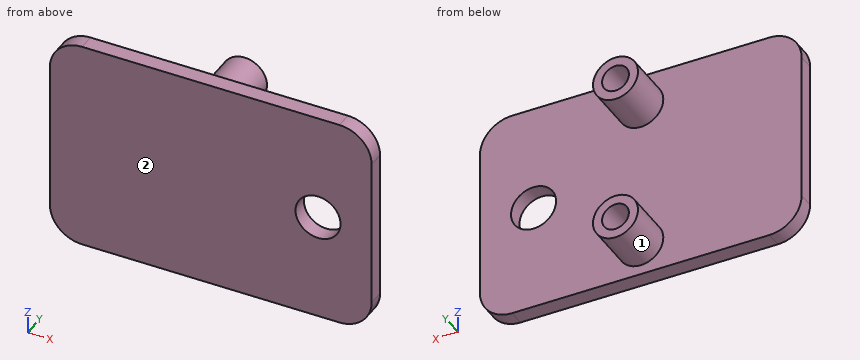
```python
from build123d import *

# Parameters (mm, degrees)
SKETCH_1_R             = 2.1
SM_BASE_FLANGE_1_DEPTH = 1.5
SKETCH_2_R             = 2.1
EXTRUDE_1_DEPTH        = 4.5
HOLE_WIZARD_M3_1_D     = 2.5
HOLE_WIZARD_M3_1_DEPTH = 4


# Sheet-metal steps are written as plain solids
with BuildPart() as part:
    # Sketch 1 → 基体-法兰1 (new body)
    with BuildSketch(Plane(origin=(0, 0, 0), x_dir=(1, 0, 0), z_dir=(0, 1, 0))):
        with BuildLine():
            Line((-7.384325118, 10), (16.615674882, 10))
            ThreePointArc((16.615674882, 10), (18.736995226, 9.121320344), (19.615674882, 7))
            Line((19.615674882, 7), (19.615674882, -7))
            ThreePointArc((19.615674882, -7), (18.736995226, -9.121320344), (16.615674882, -10))
            Line((16.615674882, -10), (-7.384325118, -10))
            ThreePointArc((-7.384325118, -10), (-9.505645461, -9.121320344), (-10.384325118, -7))
            Line((-10.384325118, -7), (-10.384325118, 7))
            ThreePointArc((-10.384325118, 7), (-9.505645461, 9.121320344), (-7.384325118, 10))
        make_face()
        with Locations(Location((14.615674882, 0, 0), (0, 0, 270))):
            Circle(SKETCH_1_R, mode=Mode.SUBTRACT)
    extrude(amount=-SM_BASE_FLANGE_1_DEPTH)

    # Sketch 2 → 凸台-拉伸1 (add)
    with BuildSketch(Plane(origin=(0, 0, 0), x_dir=(1, 0, 0), z_dir=(0, 1, 0))):
        with Locations(Location((4.615674882, 7, 0), (0, 0, 270))):
            Circle(SKETCH_2_R)
        with Locations(Location((4.615674882, -7, 0), (0, 0, 270))):
            Circle(SKETCH_2_R)
    extrude(amount=EXTRUDE_1_DEPTH)

    # M3 螺纹孔1
    with Locations(Plane(origin=(0, 4.5, 0), x_dir=(1, 0, 0), z_dir=(0, 1, 0))):
        with Locations((4.615674882, 7), (4.615674882, -7)):
            Hole(HOLE_WIZARD_M3_1_D / 2, depth=HOLE_WIZARD_M3_1_DEPTH)


solid = part.part
```
Work out the finished part from the listing and answer in its coordinate system (mm). Face numbers are marked on the shaded views. Give positions to 0.01 mm unless a question says otherwise; leave off trailing zeros. Loops run counter-clockwise (first coordinate to the right, second up) from the corner with the lowest first, then second, coordinate; pieces in that order, holes last. Notation, with made-up numbers: (-7, -11) -> (22, -11) arc R34 cw to (22, 23) -> close; hole circle Ø5 at (-27.5, 13.5). An arc over 180 degrees is marked (long way). Put each result on its own line as item: value. Start each with the question number.
Item 1: The part is cut by section B-B (y = -0.8). Give the vertices of the cut face in (x, z).
Item 2: Find the intervals of material crossed by L1, parallel to X at y = -0.3, z = 0; L2, parallel to X at y = 3.7, z = 7; L3, parallel to Y at x = -7, z = -5.25, in increasing order. Write a range as [from, to].
Item 3: The part is cut by section C-C (x = -2.25). Give the vertices of the cut face in (y, z).
Item 4: The mould has two halves that part along Z. Classify the marked faces 1 and 2: released by +Z, released by -Z, zero draft, split by the parting line, or undercut.
Item 5: The part is cut by section A-A (z = 0). Give the vertices of the cut face in (x, y), then the cut area to 3 significant figures.
Item 6: The part is cut by section D-D (y = 3.2). Give the vertices of the cut face in (x, z), then the cut area to 3 significant figures.
Item 7: Each of these flat-tipped pins is pushed along its axis until it touches: P1, Ø4, axis at x = 14.62, z = 0, coming from the +Y side; P2, Ø0.8, axis at x = 5, z = -6.5, coming from the +Y side; P3, Ø2, axis at x = 6, y = 2, coming from the +Z side. Where does it stop, or does it pass through?
Answers below:
1. outline: (-10.38, -7) arc R3 ccw to (-7.38, -10) -> (16.62, -10) arc R3 ccw to (19.62, -7) -> (19.62, 7) arc R3 ccw to (16.62, 10) -> (-7.38, 10) arc R3 ccw to (-10.38, 7) -> close; hole circle Ø4.2 at (14.62, 0)
2. L1: [-10.38, 12.52], [16.72, 19.62]
2. L2: [2.52, 3.37], [5.87, 6.72]
2. L3: [-1.5, 0]
3. outline: (-1.5, -10) -> (0, -10) -> (0, 10) -> (-1.5, 10) -> close
4. face 1: undercut
4. face 2: zero draft
5. outline: (-10.38, -1.5) -> (12.52, -1.5) -> (12.52, 0) -> (-10.38, 0) -> close; (16.72, -1.5) -> (19.62, -1.5) -> (19.62, 0) -> (16.72, 0) -> close
5. area: 38.7 mm2
6. outline: circle Ø4.2 at (4.62, -7); circle Ø4.2 at (4.62, 7); hole circle Ø2.5 at (4.62, -7); hole circle Ø2.5 at (4.62, 7)
6. area: 17.9 mm2
7. P1: through
7. P2: y = 0.5
7. P3: z = 9.06
